from build123d import *

# Parameters (mm, degrees)
SKETCH1_W               = 180
SKETCH1_H               = 250
BOSS_EXTRUDE1_DEPTH     = 7
FILLET1_R               = 5
SKETCH4_R               = 1.73
CUT_EXTRUDE2_DEPTH      = 7
MIRROR4_COPY_1_SKETCH_R = 1.73
MIRROR4_COPY_1_DEPTH    = 7
SKETCH6_R               = 1.73
CUT_EXTRUDE3_DEPTH      = 7
MIRROR7_COPY_1_SKETCH_R = 1.73
MIRROR7_COPY_1_DEPTH    = 7
SKETCH7_R               = 1.73
CUT_EXTRUDE5_DEPTH      = 7
CUT_EXTRUDE8_DEPTH      = 7
SKETCH10_W              = 4
SKETCH10_H              = 7
CUT_EXTRUDE14_DEPTH     = 7
SKETCH10_9_W            = 4
SKETCH10_9_H            = 22
CUT_EXTRUDE15_DEPTH     = 7
SKETCH10_10_W           = 4
SKETCH10_10_H           = 22
CUT_EXTRUDE16_DEPTH     = 7
SKETCH10_11_W           = 4
SKETCH10_11_H           = 12
CUT_EXTRUDE17_DEPTH     = 7
SKETCH16_R              = 1.73
CUT_EXTRUDE18_DEPTH     = 7
SKETCH17_R              = 1.73
CUT_EXTRUDE19_DEPTH     = 7


with BuildPart() as part:
    # Sketch1 → Boss-Extrude1 (new body)
    with BuildSketch(Plane.XY):
        Rectangle(SKETCH1_W, SKETCH1_H)
    extrude(amount=BOSS_EXTRUDE1_DEPTH)

    # Fillet1
    fillet1_edges = [part.edges().sort_by_distance(p)[0] for p in [
        (90, -125, 3.5),
        (-90, -125, 3.5),
        (-90, 125, 3.5),
        (90, 125, 3.5),
    ]]
    fillet(fillet1_edges, radius=FILLET1_R)

    # Sketch4 → Cut-Extrude2 (cut)
    with BuildSketch(Plane(origin=(0, 0, 0), x_dir=(-1, 0, 0), z_dir=(0, 0, -1))):
        with Locations((-59.94, 94.96)):
            Circle(SKETCH4_R)
        with Locations((-84, 94.96)):
            Circle(SKETCH4_R)
        with Locations((-84, 65.04)):
            Circle(SKETCH4_R)
        with Locations((-59.94, 65.04)):
            Circle(SKETCH4_R)
    cut_extrude2 = extrude(amount=-CUT_EXTRUDE2_DEPTH, mode=Mode.SUBTRACT)

    # Mirror3: Cut-Extrude2 across plane
    add(cut_extrude2.mirror(Plane(origin=(0, 0, 0), x_dir=(0, 0, 1), z_dir=(1, 0, 0))), mode=Mode.SUBTRACT)

    # Mirror4: Cut-Extrude2 across plane
    add(cut_extrude2.mirror(Plane.ZX), mode=Mode.SUBTRACT)

    # Mirror4 copy 1 sketch → Mirror4 copy 1 (cut)
    with BuildSketch(Plane(origin=(0, 0, 0), x_dir=(1, 0, 0), z_dir=(0, 0, -1))):
        with Locations((-59.94, 94.96)):
            Circle(MIRROR4_COPY_1_SKETCH_R)
        with Locations((-84, 94.96)):
            Circle(MIRROR4_COPY_1_SKETCH_R)
        with Locations((-84, 65.04)):
            Circle(MIRROR4_COPY_1_SKETCH_R)
        with Locations((-59.94, 65.04)):
            Circle(MIRROR4_COPY_1_SKETCH_R)
    extrude(amount=-MIRROR4_COPY_1_DEPTH, mode=Mode.SUBTRACT)

    # Sketch6 → Cut-Extrude3 (cut)
    with BuildSketch(Plane(origin=(0, 0, 0), x_dir=(-1, 0, 0), z_dir=(0, 0, -1))):
        with Locations((61.71, -13.64)):
            Circle(SKETCH6_R)
        with Locations((15.99, -13.64)):
            Circle(SKETCH6_R)
        with Locations((15.99, -49.2)):
            Circle(SKETCH6_R)
        with Locations((61.71, -49.2)):
            Circle(SKETCH6_R)
    cut_extrude3 = extrude(amount=-CUT_EXTRUDE3_DEPTH, mode=Mode.SUBTRACT)

    # Mirror5: Cut-Extrude3 across plane
    add(cut_extrude3.mirror(Plane(origin=(0, 0, 0), x_dir=(0, 0, 1), z_dir=(1, 0, 0))), mode=Mode.SUBTRACT)

    # Mirror7: Cut-Extrude3 across plane
    add(cut_extrude3.mirror(Plane.ZX), mode=Mode.SUBTRACT)

    # Mirror7 copy 1 sketch → Mirror7 copy 1 (cut)
    with BuildSketch(Plane(origin=(0, 0, 0), x_dir=(1, 0, 0), z_dir=(0, 0, -1))):
        with Locations((61.71, -13.64)):
            Circle(MIRROR7_COPY_1_SKETCH_R)
        with Locations((15.99, -13.64)):
            Circle(MIRROR7_COPY_1_SKETCH_R)
        with Locations((15.99, -49.2)):
            Circle(MIRROR7_COPY_1_SKETCH_R)
        with Locations((61.71, -49.2)):
            Circle(MIRROR7_COPY_1_SKETCH_R)
    extrude(amount=-MIRROR7_COPY_1_DEPTH, mode=Mode.SUBTRACT)

    # Sketch7 → Cut-Extrude5 (cut)
    with BuildSketch(Plane(origin=(0, 0, 0), x_dir=(-1, 0, 0), z_dir=(0, 0, -1))):
        with Locations((-9.635797548, 8.125)):
            Circle(SKETCH7_R)
        with Locations((10.22, -8.125)):
            Circle(SKETCH7_R)
        with Locations((-39.835797548, -8.125)):
            Circle(SKETCH7_R)
        with Locations((40.42, 8.125)):
            Circle(SKETCH7_R)
    extrude(amount=-CUT_EXTRUDE5_DEPTH, mode=Mode.SUBTRACT)

    # Sketch9 → Cut-Extrude8 (cut)
    with BuildSketch(Plane(origin=(0, 0, 0), x_dir=(-1, 0, 0), z_dir=(0, 0, -1))):
        Polygon((74, 0), (74, 17), (66, 17), (66, -17), (74, -17), align=None)
        Polygon((60, 0), (60, 3), (48, 3), (48, -3), (60, -3), align=None)
    cut_extrude8 = extrude(amount=-CUT_EXTRUDE8_DEPTH, mode=Mode.SUBTRACT)

    # Mirror9: Cut-Extrude8 across plane
    add(cut_extrude8.mirror(Plane(origin=(0, 0, 0), x_dir=(0, 0, 1), z_dir=(1, 0, 0))), mode=Mode.SUBTRACT)

    # Sketch10 → Cut-Extrude14 (cut)
    with BuildSketch(Plane.XY.offset(7)):
        with Locations((76, 111.5)):
            Rectangle(SKETCH10_W, SKETCH10_H)
    cut_extrude14 = extrude(amount=-CUT_EXTRUDE14_DEPTH, mode=Mode.SUBTRACT)

    # Sketch10<9> → Cut-Extrude15 (cut)
    with BuildSketch(Plane.XY.offset(7)):
        with Locations((76, 40)):
            Rectangle(SKETCH10_9_W, SKETCH10_9_H)
    cut_extrude15 = extrude(amount=-CUT_EXTRUDE15_DEPTH, mode=Mode.SUBTRACT)

    # Sketch10<10> → Cut-Extrude16 (cut)
    with BuildSketch(Plane.XY.offset(7)):
        with Locations((76, -40)):
            Rectangle(SKETCH10_10_W, SKETCH10_10_H)
    cut_extrude16 = extrude(amount=-CUT_EXTRUDE16_DEPTH, mode=Mode.SUBTRACT)

    # Sketch10<11> → Cut-Extrude17 (cut)
    with BuildSketch(Plane.XY.offset(7)):
        with Locations((76, -114)):
            Rectangle(SKETCH10_11_W, SKETCH10_11_H)
    cut_extrude17 = extrude(amount=-CUT_EXTRUDE17_DEPTH, mode=Mode.SUBTRACT)

    # Mirror11: Cut-Extrude14, Cut-Extrude15, Cut-Extrude16, Cut-Extrude17 across plane
    add(cut_extrude14.mirror(Plane(origin=(0, 0, 0), x_dir=(0, 0, 1), z_dir=(1, 0, 0))), mode=Mode.SUBTRACT)
    add(cut_extrude15.mirror(Plane(origin=(0, 0, 0), x_dir=(0, 0, 1), z_dir=(1, 0, 0))), mode=Mode.SUBTRACT)
    add(cut_extrude16.mirror(Plane(origin=(0, 0, 0), x_dir=(0, 0, 1), z_dir=(1, 0, 0))), mode=Mode.SUBTRACT)
    add(cut_extrude17.mirror(Plane(origin=(0, 0, 0), x_dir=(0, 0, 1), z_dir=(1, 0, 0))), mode=Mode.SUBTRACT)

    # Sketch16 → Cut-Extrude18 (cut)
    with BuildSketch(Plane.XY.offset(7)):
        with Locations((84, -112)):
            Circle(SKETCH16_R)
        with Locations((84, -52)):
            Circle(SKETCH16_R)
        with Locations((84, 23)):
            Circle(SKETCH16_R)
        with Locations((84, 56)):
            Circle(SKETCH16_R)
    cut_extrude18 = extrude(amount=-CUT_EXTRUDE18_DEPTH, mode=Mode.SUBTRACT)

    # Mirror12: Cut-Extrude18 across plane
    add(cut_extrude18.mirror(Plane(origin=(0, 0, 0), x_dir=(0, 0, 1), z_dir=(1, 0, 0))), mode=Mode.SUBTRACT)

    # Sketch17 → Cut-Extrude19 (cut)
    with BuildSketch(Plane(origin=(0, 0, 0), x_dir=(-1, 0, 0), z_dir=(0, 0, -1))):
        with Locations((0, -97.16)):
            Circle(SKETCH17_R)
        with Locations((0, -38.66)):
            Circle(SKETCH17_R)
        with Locations((0, 97.16)):
            Circle(SKETCH17_R)
        with Locations((0, 38.66)):
            Circle(SKETCH17_R)
    extrude(amount=-CUT_EXTRUDE19_DEPTH, mode=Mode.SUBTRACT)


solid = part.part
Design review of the part built by this model. Coordinates are the model's own, in mm. A direction names the side the tool comes from. Round coordinates to 2 decimals unless told otherwise and drop trailing zeros. One line per question, with ' | ' between items.
(1) Take a section at A-A, the plane z = 5.25. State how many separate pieces and enclosed holes the cut face has, and give its area (3 significant figures).
Result sheet:
separate pieces: 1 | enclosed holes: 60 | area: 43,300 mm2
(2) Wall thickness on line 1 (X direction, y = -35.5, z = 6.5); line 2 (Y direction, x = 0, z = 4); line 3 (X direction, y = -6, z = 1.75): over which ranges is each line inside the solid? List them lowest first. Write a range as [from, to].
Result sheet:
line 1: [-90, -78], [-74, 74], [78, 90] | line 2: [-125, -98.89], [-95.43, -40.39], [-36.93, 36.93], [40.39, 95.43], [98.89, 125] | line 3: [-90, -74], [-66, 66], [74, 90]
(3) Insertion check: P1, Ø3, axis at x = 61.71, y = -13.64, coming from the -Z side. The pin has a flat end and moves straight along its axis. Give the tip position at first contact, or say it passes through.
Result sheet:
P1: through
(4) Machinability: for faces 4 (the flat face through (-74, 111, 4)), 5 (the flat face through (-1, 2, 7)), which of the approach directions +Z, -Z, +X, -X, +Y, -Y give a long, thin tool a straight path to every point of the face, cutting with its end or side? Answer none if there is none.
Result sheet:
face 4: +Z, -Z | face 5: +Z, +X, -X, +Y, -Y
(5) Draft analysis for pull direction Y (two halves, no side actions). For faces 1 (the flat face through (-90, -2, 3)), 2 (the cylindrical face through (-89, -123, 4)), 3 (the flat face through (-54, 3, 3)), state which applies: released by +Y, released by -Y, zero draft, split by the parting line, or undercut.
Result sheet:
face 1: zero draft | face 2: released by -Y | face 3: undercut
